Input: dimensioned drawing with shaded views. Units: mm. Origin: part minimum x, y, z. A direction names the side the tool comes from. Round coordinates to 2 decimals unless told otherwise and drop trailing zeros. Write each loop counter-clockwise with the first axis right and the second up, starting at its lowest first coordinate (ties: lowest second). Pieces come first, ordered by that corner, then holes. Notation, with made-up numbers: M 65.25,19.25 L 83.25,19.25 A20 ccw 83.25,53.25 Z; hole C 33,29 d2. An arc over 180 degrees is marked long. Answer as CSV lines item,"result". Start each with the question number.
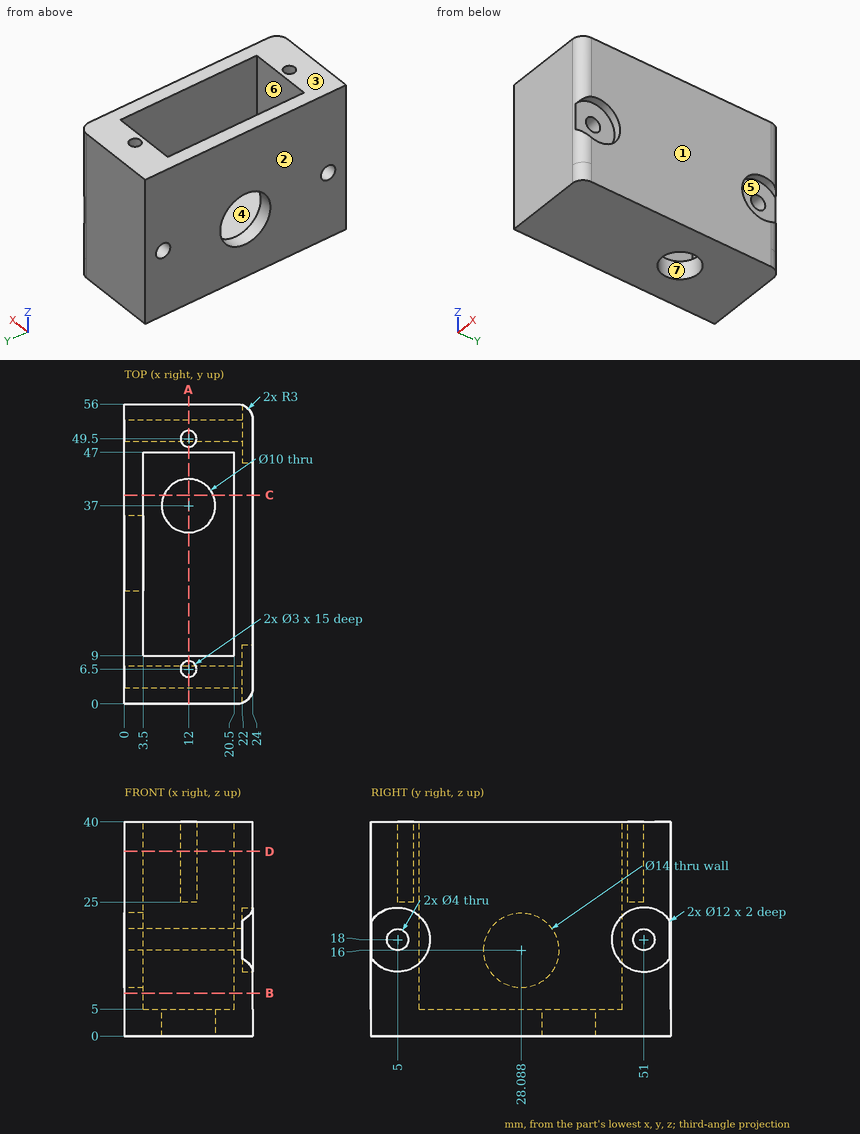
Item 1: Cut plane A-A, the plane x = 12. Return loops of the section in (y, z).
Item 2: Line query: line 1 (Y direction, x = 12, z = 32.25); line 2 (Y direction, x = 14.25, z = 7.5); line 3 (Z direction, x = 9.25, y = 51). Output: solid intervals per line, ascending. Write a range as [from, to].
Item 3: Cut plane D-D, the plane z = 34.5. Return loops of the section in (x, y), plus the area to 3 significant figures.
Item 4: Access query for the marked faces 5, 6 and 7. Directions: +Z, -Z, +X, -X, +Y, -Y. A direction counts if a zero-diameter tool reaches every point of the face in a straight line with its end or side. Return the directions, or none.
Item 5: Cut plane B-B, the plane z = 8. Return loops of the section in (x, y).
Item 6: Cut plane C-C, the plane y = 39. Return loops of the section in (x, z), plus the area to 3 significant figures.
Item 7: Pin query (flat end, axial travel): pin 1 Ø0.9 at (x, y) = (12.5, 6.5) entering from +Z; pin 2 Ø8.5 at (x, y) = (9, 22.5) entering from +Z; pin 3 Ø5.5 at (y, z) = (3.5, 19) entering from +X. Return the tip coordinate at first contact, or that it passes through.
Item 8: Draft query along X for the marked faces 1, 2, 3 and 4. Return one class per face: +X half, -X half, draft (parallel to the pull), parting line (faces both ways), or undercut.
Results list:
1,outline,"M 0,0 L 32,0 L 32,5 L 9,5 L 9,40 L 8,40 L 8,25 L 5,25 L 5,40 L 0,40 Z; M 42,0 L 56,0 L 56,40 L 51,40 L 51,25 L 48,25 L 48,40 L 47,40 L 47,5 L 42,5 Z; hole C 5,18 d4; hole C 51,18 d4"
2,line 1,"[0, 5], [8, 9], [47, 48], [51, 56]"
2,line 2,"[0, 9], [47, 56]"
2,line 3,"[0, 16], [20, 40]"
3,outline,"M 0,0 L 21,0 A3 ccw 24,3 L 24,53 A3 ccw 21,56 L 0,56 Z; hole M 3.5,9 L 20.5,9 L 20.5,47 L 3.5,47 Z; hole C 12,6.5 d3; hole C 12,49.5 d3"
3,area,"680 mm²"
4,face 5,"+X"
4,face 6,"+Z"
4,face 7,"+Z, -Z"
5,outline,"M 0,0 L 21,0 A3 ccw 24,3 L 24,53 A3 ccw 21,56 L 0,56 Z; hole M 3.5,9 L 20.5,9 L 20.5,47 L 3.5,47 Z"
6,outline,"M 0,0 L 7.42,0 L 7.42,5 L 3.5,5 L 3.5,40 L 0,40 Z; M 16.58,0 L 24,0 L 24,40 L 20.5,40 L 20.5,5 L 16.58,5 Z"
6,area,"319 mm²"
7,pin 1,"z = 25"
7,pin 2,"z = 5"
7,pin 3,"x = 22"
8,face 1,"+X half"
8,face 2,"-X half"
8,face 3,"draft"
8,face 4,"undercut"
